```python
from build123d import *

# Parameters (mm, degrees)
SKETCH2_R           = 1.5
BOSS_EXTRUDE1_DEPTH = 3.75


with BuildPart() as part:
    # Sketch1 → Revolve1 (revolve)
    with BuildSketch(Plane.XY, mode=Mode.PRIVATE) as revolve1_sk:
        Polygon((0, 0), (0, 22), (0.5, 22), (2.5, 24), (3.2, 24), (3.2, 22), (2.40945179, 22), (2, 21), (2, 0), align=None)
    revolve(revolve1_sk.sketch.rotate(Axis((0, 0, 0), (0, 1, 0)), 90), axis=Axis((0, 0, 0), (0, 1, 0)))

    # Sketch2 → Boss-Extrude1 (add, symmetric)
    with BuildSketch(Plane.XY):
        with Locations((0, 24)):
            Circle(SKETCH2_R)
    extrude(amount=BOSS_EXTRUDE1_DEPTH, both=True)


solid = part.part
```
Can you work these out from the model? Positions are in its coordinate system, mm. A direction names the side the tool comes from. Give positions to 0.01 mm unless a question says otherwise; leave off trailing zeros. Order: outer loops, then holes, each group sorted by start corner. A loop starts at its lowest first (then second) coordinate and runs counter-clockwise, first axis right, second up. Notation, with made-up numbers: M -17.5,44 L 33.5,44 A29 ccw 33.5,82 Z; hole C 42.5,59.5 d11. An arc over 180 degrees is marked long. Write item = value, one per line. Start each with the question number.
Q1. For faces 4 (the flat face through (3, 24, 0)), 5 (the cylindrical face through (1.947, 22.986, 2.539)), 6 (the flat face through (0, 22, 0)), which set-ups out of +Z, -Z, +X, -X, +Y, -Y let a thin tool reach every point of the face, with its end or its side?
Q2. Suppose I cut it at D-D (y = 24.25). Write out the boundary of the cut face in (x, z).
Q3. Suppose I cut it at B-B (x = 0). Write out the boundary of the cut face in (y, z), plus the area to 3 significant figures.
Q4. Suppose I cut it at A-A (z = 0). Write out the boundary of the cut face in (x, y).
Q5. Suppose I cut it at C-C (y = 4.5). Write out the boundary of the cut face in (x, z).
Q6. I need wall thicknesses on probe 1 along Y at (x, z) = (-0.25, -0.75); probe 2 along X at (y, z) = (9.5, 0); probe 3 along Y at (x, z) = (1.75, -2.5). Which ranges of each line are inside material? Lowest first, please. Write a range as [from, to].
Q7. We'd pull the mould along Z, two halves only. Please class faces 1 (the flat face through (-3, 24, 0)), 2 (the conical face through (-0.53, 22.13, -0.34)), 3 (the cylindrical face through (2, 10, 0)): pulls with the +Z half, pulls with the -Z half, needs draft (parallel to the pull), parting line crosses it, or undercut.
Q8. Will these pins go through, and if not, where does the flat tip stop? pin 1 Ø1.5 at (x, y) = (0, 4) entering from -Z; pin 2 Ø1.5 at (x, y) = (-2.5, 20) entering from +Z; pin 3 Ø1 at (x, z) = (-2, -0.5) entering from -Y; pin 4 Ø0.9 at (x, z) = (2.5, 0) entering from +Y.
Check result:
q1.face_4 = +Z, -Z, +X, +Y
q1.face_5 = -Y
q1.face_6 = none
q2.outline = M -1.48,-3.75 L 1.48,-3.75 L 1.48,3.75 L -1.48,3.75 Z
q3.outline = M 0,-2 L 21,-2 L 22,-2.41 L 22,-3.2 L 22.5,-3.2 L 22.5,-3.75 L 25.5,-3.75 L 25.5,3.75 L 22.5,3.75 L 22.5,3.2 L 22,3.2 L 22,2.41 L 21,2 L 0,2 Z; hole M 22,-0.5 L 22.5,-1 L 22.5,1 L 22,0.5 Z
q3.area = 113 mm2
q4.outline = M -3.2,22 L -2.41,22 L -2,21 L -2,0 L 2,0 L 2,21 L 2.41,22 L 3.2,22 L 3.2,24 L 2.5,24 L 0.5,22 L -0.5,22 L -2.5,24 L -3.2,24 Z; C 0,24 d3
q5.outline = C 0,0 d4
q6.probe_1 = [0, 22.29], [22.52, 25.48]
q6.probe_2 = [-2, 2]
q6.probe_3 = [22, 24]
q7.face_1 = needs draft
q7.face_2 = undercut
q7.face_3 = parting line crosses it
q8.pin_1 = -2
q8.pin_2 = 0.97
q8.pin_3 = 0
q8.pin_4 = 24
